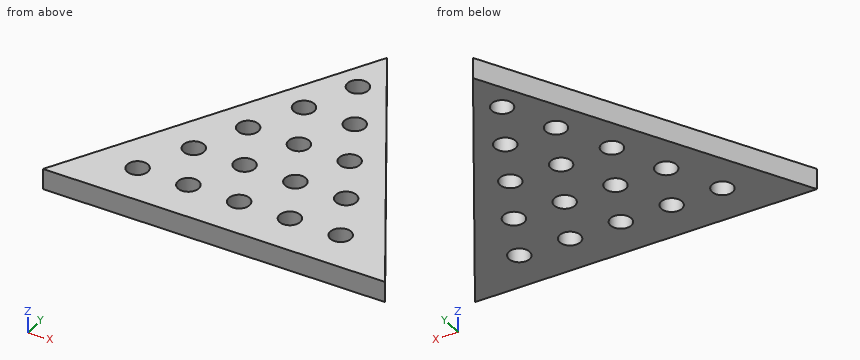
from build123d import *

# Parameters (mm, degrees)
F7_DEPTH = 6.35
F5_R     = 3.175
F1_R     = 3.175
F2_R     = 3.175
F3_R     = 3.175
F4_R     = 3.175
F8_DEPTH = 6.35


with BuildPart() as f7:
    # F6 (on face) → F7 (new body)
    with BuildSketch(Plane.XY):
        Polygon((-8.272192, 0), (94.380685, 0), (43.054246, 88.9), align=None)
    extrude(amount=F7_DEPTH)

    # F5 (on face) + F1 (on face) + F2 (on face) + F3 (on face) + F4 (on face) → F8 (cut, through all)
    with BuildSketch(Plane.XY):
        with Locations((43.2308, 73.655994)):
            Circle(F5_R)
    with BuildSketch(Plane.XY):
        with Locations((12.7, 12.7)):
            Circle(F1_R)
        with Locations((27.94, 12.7)):
            Circle(F1_R)
        with Locations((43.18, 12.7)):
            Circle(F1_R)
        with Locations((58.42, 12.7)):
            Circle(F1_R)
        with Locations((73.66, 12.7)):
            Circle(F1_R)
    with BuildSketch(Plane.XY):
        with Locations((20.669391, 27.935994)):
            Circle(F2_R)
        with Locations((35.909391, 27.935994)):
            Circle(F2_R)
        with Locations((51.149391, 27.935994)):
            Circle(F2_R)
        with Locations((66.389391, 27.935994)):
            Circle(F2_R)
    with BuildSketch(Plane.XY):
        with Locations((28.076159, 43.175994)):
            Circle(F3_R)
        with Locations((43.316159, 43.175994)):
            Circle(F3_R)
        with Locations((58.556159, 43.175994)):
            Circle(F3_R)
    with BuildSketch(Plane.XY):
        with Locations((35.941, 58.415994)):
            Circle(F4_R)
        with Locations((51.181, 58.415994)):
            Circle(F4_R)
    extrude(amount=F8_DEPTH, mode=Mode.SUBTRACT)


solid = f7.part
Verification items for the finished model (mm, model axes). Give positions to 0.01 mm unless a question says otherwise; leave off trailing zeros. Loops run counter-clockwise (first coordinate to the right, second up) from the corner with the lowest first, then second, coordinate; pieces in that order, holes last. Notation, with made-up numbers: (86, 16) - (105, 16) arc R11 cw to (105, 31) - close; hole circle Ø4 at (77, 23.25). An arc over 180 degrees is marked (long way). Write item = value, one per line. Start each with the question number.
Q1. Cross-section at D-D, the plane x = 11. Enter the section's corners in (y, z), and give its area (3 significant figures).
Q2. Thickness scan on line 1 (Y direction, x = 58.42, z = 2) (3 decimals); line 2 (Y direction, x = 54, z = 2.75); line 3 (X direction, y = 46, z = 5.75). Record the ranges inside material, lowest first.
Q3. Cross-section at C-C, the plane y = 12.7. Enter the section's corners in (x, z) (3 decimals), and give its area (3 significant figures).
Q4. Depth check by flat-ended pin: P1, Ø5, axis at x = 43.18, y = 12.7, coming from the +Z side; P2, Ø1.5, axis at y = 79, z = 3.5, coming from the -X side. Enter the tip coordinate at first touch or a pass-through.
Q5. Cross-section at B-B, the plane z = 3.75. State how many separate pieces and enclosed holes the cut face has, and give its area (3 significant figures).
Q6. Cross-section at A-A, the plane x = 57.5. Enter the section's corners in (y, z).
Answer key:
q1.outline = (0, 0) - (10.02, 0) - (10.02, 6.35) - (0, 6.35) - close; (15.38, 0) - (33.38, 0) - (33.38, 6.35) - (15.38, 6.35) - close
q1.area = 178 mm^2
q2.line_1 = 0 to 9.525, 15.875 to 40.004, 46.348 to 62.286
q2.line_2 = 0 to 26.54, 29.33 to 56.96, 59.88 to 69.94
q2.line_3 = 18.29 to 26.63, 29.53 to 41.87, 44.77 to 57.11, 60.01 to 67.82
q3.outline = (-0.94, 0) - (9.525, 0) - (9.525, 6.35) - (-0.94, 6.35) - close; (15.875, 0) - (24.765, 0) - (24.765, 6.35) - (15.875, 6.35) - close; (31.115, 0) - (40.005, 0) - (40.005, 6.35) - (31.115, 6.35) - close; (46.355, 0) - (55.245, 0) - (55.245, 6.35) - (46.355, 6.35) - close; (61.595, 0) - (70.485, 0) - (70.485, 6.35) - (61.595, 6.35) - close; (76.835, 0) - (87.048, 0) - (87.048, 6.35) - (76.835, 6.35) - close
q3.area = 357 mm^2
q4.P1 = through
q4.P2 = 36.91
q5.separate_pieces = 1
q5.enclosed_holes = 15
q5.area = 4,090 mm^2
q6.outline = (0, 0) - (9.66, 0) - (9.66, 6.35) - (0, 6.35) - close; (15.74, 0) - (40.18, 0) - (40.18, 6.35) - (15.74, 6.35) - close; (46.17, 0) - (63.88, 0) - (63.88, 6.35) - (46.17, 6.35) - close
